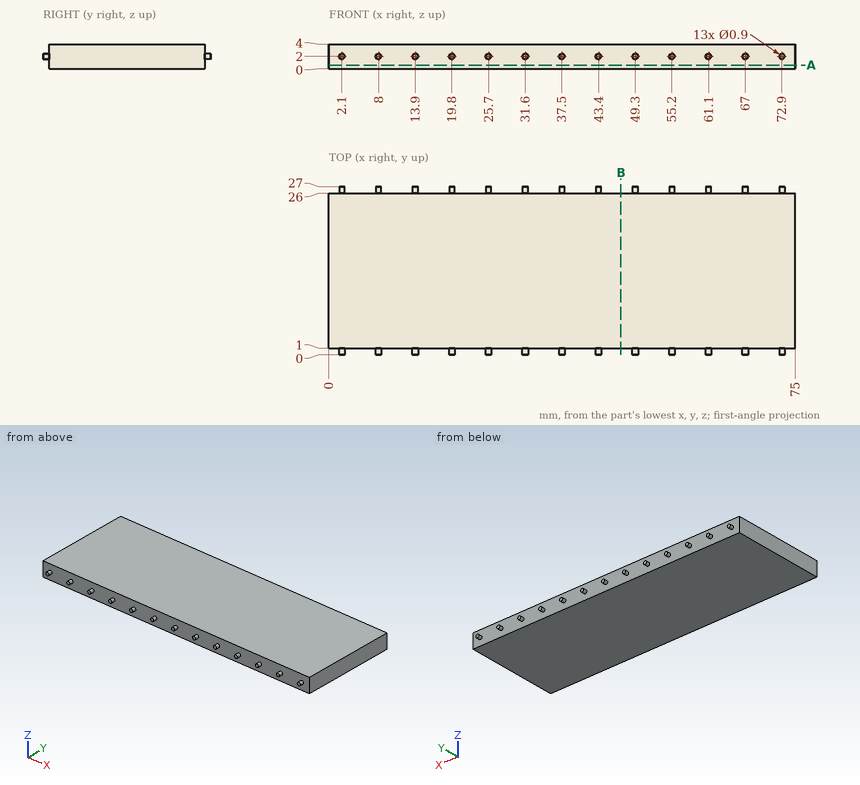
Could you check a few things on this drawing? It's one solid part, dimensions in mm from its lowest x, y, z. Give positions to 0.01 mm unless a question says otherwise; leave off trailing zeros. Write each loop counter-clockwise with the first axis right and the second up, starting at its lowest first coordinate (ties: lowest second). Pieces come first, ordered by that corner, then holes. Notation, with made-up numbers: (72, 84) -> (81, 84) arc R19 cw to (81, 96) -> close; hole circle Ø2 at (-31.75, 35). An arc over 180 degrees is marked (long way). Write item = value, one per line.
(1) I'm going to push flat-ended pins straight in: P1, Ø3, axis at x = 32, y = 11.5, coming from the -Z side; P2, Ø1, axis at x = 28, z = 3, coming from the +Y side. Where does each tip first touch, or does it pass through?
Worked out:
P1 = 0
P2 = 26
(2) I need wall thicknesses on probe 1 along Y at (x, z) = (45, 1.8). Which ranges of the line are inside material? Lowest first, please. Write a range as from..to.
Worked out:
probe_1 = 1..26
(3) Suppose I cut it at A-A on z = 0.6. Write out the boundary of the cut face in (x, y), then the cut area to 4 significant figures.
Worked out:
outline = (0, 1) -> (75, 1) -> (75, 26) -> (0, 26) -> close
area = 1,875 mm^2
(4) Suppose I cut it at B-B on x = 47. Write out the boundary of the cut face in (y, z), then the cut area to 3 significant figures.
Worked out:
outline = (1, 0) -> (26, 0) -> (26, 4) -> (1, 4) -> close
area = 100 mm^2
